Geometry: final body of the model. Coordinates: model frame, mm. Face numbers are marked on the shaded views. Give positions to 0.01 mm unless a question says otherwise; leave off trailing zeros. Loops run counter-clockwise (first coordinate to the right, second up) from the corner with the lowest first, then second, coordinate; pieces in that order, holes last. Notation, with made-up numbers: (81.25, 70) - (110.25, 70) arc R15 cw to (110.25, 79) - close; hole circle Ø7 at (33, 57). An arc over 180 degrees is marked (long way). Answer in a Markdown table with one row per item.
from build123d import *

# Parameters (mm, degrees)
SKETCH1_W           = 55.1
SKETCH1_H           = 55.1
BOSS_EXTRUDE1_DEPTH = 5
FILLET1_R           = 7.5
SKETCH2_R           = 3.25
CUT_EXTRUDE1_DEPTH  = 6
SKETCH3_R           = 2.5
CUT_EXTRUDE2_DEPTH  = 5
SKETCH4_R           = 4.75
CUT_EXTRUDE3_DEPTH  = 3


with BuildPart() as part:
    # Sketch1 → Boss-Extrude1 (new body)
    with BuildSketch(Plane(origin=(0, 0, 0), x_dir=(1, 0, 0), z_dir=(0, 1, 0))):
        Rectangle(SKETCH1_W, SKETCH1_H)
    extrude(amount=BOSS_EXTRUDE1_DEPTH)

    # Fillet1
    fillet1_edges = [part.edges().sort_by_distance(p)[0] for p in [
        (27.55, 2.5, 27.55),
        (-27.55, 2.5, 27.55),
        (-27.55, 2.5, -27.55),
        (27.55, 2.5, -27.55),
    ]]
    fillet(fillet1_edges, radius=FILLET1_R)

    # Sketch2 → Cut-Extrude1 (cut, through all)
    with BuildSketch(Plane(origin=(0, 5, 0), x_dir=(1, 0, 0), z_dir=(0, 1, 0))):
        with Locations((-20.874050615, 20.870277104)):
            Circle(SKETCH2_R)
        with Locations((-20.874050615, -20.869722896)):
            Circle(SKETCH2_R)
        with Locations((20.865949385, 20.870277104)):
            Circle(SKETCH2_R)
        with Locations((20.865949385, -20.869722896)):
            Circle(SKETCH2_R)
    extrude(amount=-CUT_EXTRUDE1_DEPTH, mode=Mode.SUBTRACT)

    # Sketch3 → Cut-Extrude2 (cut)
    with BuildSketch(Plane(origin=(0, 5, 0), x_dir=(1, 0, 0), z_dir=(0, 1, 0))):
        with Locations((-10.35, 10.35)):
            Circle(SKETCH3_R)
        with Locations((10.35, 10.35)):
            Circle(SKETCH3_R)
        with Locations((-10.35, -10.35)):
            Circle(SKETCH3_R)
        with Locations((10.35, -10.35)):
            Circle(SKETCH3_R)
    extrude(amount=-CUT_EXTRUDE2_DEPTH, mode=Mode.SUBTRACT)

    # Sketch4 → Cut-Extrude3 (cut)
    with BuildSketch(Plane.XZ):
        with Locations((-10.35, 10.35)):
            Circle(SKETCH4_R)
        with Locations((10.35, 10.35)):
            Circle(SKETCH4_R)
        with Locations((10.35, -10.35)):
            Circle(SKETCH4_R)
        with Locations((-10.35, -10.35)):
            Circle(SKETCH4_R)
    extrude(amount=-CUT_EXTRUDE3_DEPTH, mode=Mode.SUBTRACT)


solid = part.part
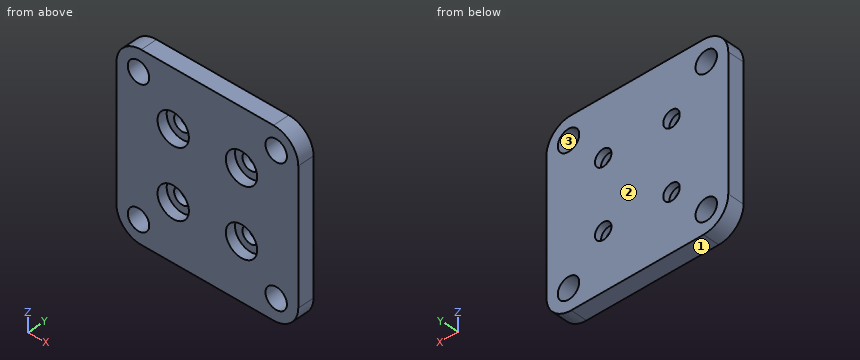
Q1. Cut plane C-C (y = 1). Give the number of separate pieces and of enclosed holes in the cut face, and give its area (3 significant figures).
Check values:
| item | result |
|---|---|
| separate pieces | 1 |
| enclosed holes | 8 |
| area | 2,570 mm² |
Q2. First-contact query: pin 1 (3 mm diameter, centred on x = -11, z = -12, fed in from -Y). Flat tip, straight axial feed; report the tip coordinate or a pass-through.
Check values:
| item | result |
|---|---|
| pin 1 | y = 3 |
Q3. Draft query along Z for the marked faces 1, 2 and 3. Return one class per face: pulls with the +Z half, pulls with the -Z half, needs draft (parallel to the pull), parting line crosses it, or undercut.
Check values:
| item | result |
|---|---|
| face 1 | pulls with the -Z half |
| face 2 | needs draft |
| face 3 | undercut |
Q4. Material intervals for line 1 along Z through (x, y) = (10.35, 1.95); line 2 along X through (y, z) = (4.5, -10.35); line 3 along X through (y, z) = (0.55, -14), sorted ascending.
Check values:
| item | result |
|---|---|
| line 1 | -27.55 to -15.1, -5.6 to 5.6, 15.1 to 27.55 |
| line 2 | -27.55 to -12.85, -7.85 to 7.85, 12.85 to 27.55 |
| line 3 | -27.55 to -13.39, -7.31 to 7.31, 13.39 to 27.55 |
Q5. Cut plane B-B (z = -10.35). Output: boundary loops of the cut face in (x, y), and give its area (4 significant figures).
Check values:
| item | result |
|---|---|
| outline | (-27.55, 0) - (-15.1, 0) - (-15.1, 3) - (-12.85, 3) - (-12.85, 5) - (-27.55, 5) - close; (-7.85, 3) - (-5.6, 3) - (-5.6, 0) - (5.6, 0) - (5.6, 3) - (7.85, 3) - (7.85, 5) - (-7.85, 5) - close; (12.85, 3) - (15.1, 3) - (15.1, 0) - (27.55, 0) - (27.55, 5) - (12.85, 5) - close |
| area | 198.5 mm² |
Q6. Cut plane D-D (x = 22). Output: boundary loops of the cut face in (y, z).
Check values:
| item | result |
|---|---|
| outline | (0, -27.29) - (5, -27.29) - (5, -23.92) - (0, -23.92) - close; (0, -17.82) - (5, -17.82) - (5, 17.82) - (0, 17.82) - close; (0, 23.92) - (5, 23.92) - (5, 27.29) - (0, 27.29) - close |
Q7. Cut plane A-A (x = 10.35). Output: boundary loops of the cut face in (y, z).
Check values:
| item | result |
|---|---|
| outline | (0, -27.55) - (5, -27.55) - (5, -12.85) - (3, -12.85) - (3, -15.1) - (0, -15.1) - close; (0, -5.6) - (3, -5.6) - (3, -7.85) - (5, -7.85) - (5, 7.85) - (3, 7.85) - (3, 5.6) - (0, 5.6) - close; (0, 15.1) - (3, 15.1) - (3, 12.85) - (5, 12.85) - (5, 27.55) - (0, 27.55) - close |
